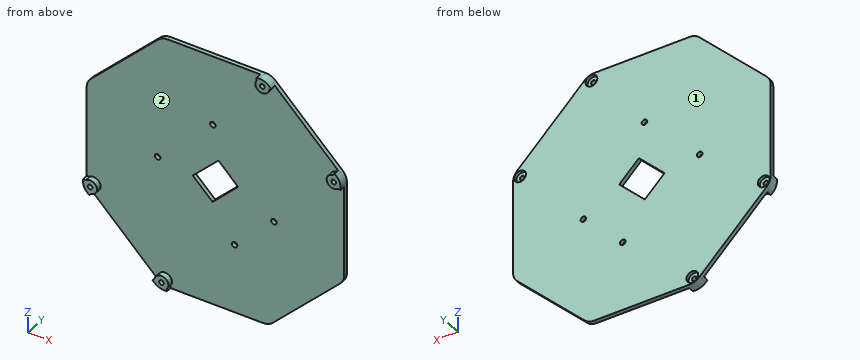
```python
from build123d import *

# Parameters (mm, degrees)
BOSS_EXTRUDE1_DEPTH                              = 3
BOSS_EXTRUDE3_DEPTH                              = 7
CBORE_FOR_M3_HEX_HEAD_MACHINE_SCREW1_D           = 3.4
CBORE_FOR_M3_HEX_HEAD_MACHINE_SCREW1_CBORE_D     = 8.4
CBORE_FOR_M3_HEX_HEAD_MACHINE_SCREW1_CBORE_DEPTH = 2.3
FILLET1_R                                        = 10
SKETCH23_R                                       = 2
CUT_EXTRUDE1_DEPTH                               = 131.843677004
CUT_EXTRUDE2_DEPTH                               = 131.843677004


with BuildPart() as part:
    # Sketch1 → Boss-Extrude1 (new body)
    with BuildSketch(Plane(origin=(0, 0, 0), x_dir=(1, 0, 0), z_dir=(0, 1, 0))):
        Polygon((92.387953251, -38.268343237), (92.387953251, 38.268343237), (38.268343237, 92.387953251), (-38.268343237, 92.387953251), (-92.387953251, 38.268343237), (-92.387953251, -38.268343237), (-38.268343237, -92.387953251), (38.268343237, -92.387953251), align=None)
    extrude(amount=BOSS_EXTRUDE1_DEPTH)

    # Sketch13 → Boss-Extrude3 (add)
    with BuildSketch(Plane(origin=(0, 3, 0), x_dir=(1, 0, 0), z_dir=(0, 1, 0))):
        with BuildLine():
            ThreePointArc((-90.387953251, 32.197275425), (-82.768555589, 34.283858263), (-86.68084647, 41.147022893))
            Line((-86.68084647, 41.147022893), (-88.095060032, 42.561236455))
            Line((-88.095060032, 42.561236455), (-92.387953251, 38.268343237))
            Line((-92.387953251, 38.268343237), (-92.387953251, 32.197275425))
            Line((-92.387953251, 32.197275425), (-90.387953251, 32.197275425))
        make_face()
        with BuildLine():
            Line((92.387953251, -32.197275425), (90.387953251, -32.197275425))
            ThreePointArc((90.387953251, -32.197275425), (82.768555589, -34.283858263), (86.68084647, -41.147022893))
            Line((86.68084647, -41.147022893), (88.095060032, -42.561236455))
            Line((88.095060032, -42.561236455), (92.387953251, -38.268343237))
            Line((92.387953251, -38.268343237), (92.387953251, -32.197275425))
        make_face()
        with BuildLine():
            Line((38.268343237, -92.387953251), (42.561236455, -88.095060032))
            Line((42.561236455, -88.095060032), (41.147022893, -86.68084647))
            ThreePointArc((41.147022893, -86.68084647), (34.283858263, -82.768555589), (32.197275425, -90.387953251))
            Line((32.197275425, -90.387953251), (32.197275425, -92.387953251))
            Line((32.197275425, -92.387953251), (38.268343237, -92.387953251))
        make_face()
        with BuildLine():
            ThreePointArc((-41.147022893, 86.68084647), (-34.283858263, 82.768555589), (-32.197275425, 90.387953251))
            Line((-32.197275425, 90.387953251), (-32.197275425, 92.387953251))
            Line((-32.197275425, 92.387953251), (-38.268343237, 92.387953251))
            Line((-38.268343237, 92.387953251), (-42.561236455, 88.095060032))
            Line((-42.561236455, 88.095060032), (-41.147022893, 86.68084647))
        make_face()
    extrude(amount=-BOSS_EXTRUDE3_DEPTH)

    # CBORE for M3 Hex Head Machine Screw1 (through all)
    with Locations(Plane(origin=(0, 3, 0), x_dir=(1, 0, 0), z_dir=(0, 1, 0))):
        with Locations((36.197275425, -87.387953251), (87.387953251, -36.197275425), (-36.197275425, 87.387953251), (-87.387953251, 36.197275425)):
            CounterBoreHole(CBORE_FOR_M3_HEX_HEAD_MACHINE_SCREW1_D / 2, CBORE_FOR_M3_HEX_HEAD_MACHINE_SCREW1_CBORE_D / 2, CBORE_FOR_M3_HEX_HEAD_MACHINE_SCREW1_CBORE_DEPTH)

    # Fillet1
    fillet1_edges = [part.edges().sort_by_distance(p)[0] for p in [
        (-92.387953251, 1.5, 38.268343237),
        (-92.387953251, -0.5, -38.268343237),
        (-38.268343237, -0.5, -92.387953251),
        (38.268343237, 1.5, -92.387953251),
        (92.387953251, 1.5, -38.268343237),
        (92.387953251, -0.5, 38.268343237),
        (38.268343237, -0.5, 92.387953251),
        (-38.268343237, 1.5, 92.387953251),
    ]]
    fillet(fillet1_edges, radius=FILLET1_R)

    # Sketch23 → Cut-Extrude1 (cut, through all)
    with BuildSketch(Plane(origin=(0, 3, 0), x_dir=(1, 0, 0), z_dir=(0, 1, 0))):
        with Locations(Location((-41.471812717, -1.87383297, 0), (0, 0, 270))):
            Circle(SKETCH23_R)
        with Locations(Location((13.682516216, 41.966787463, 0), (0, 0, 270))):
            Circle(SKETCH23_R)
        with Locations(Location((41.966787463, 13.682516216, 0), (0, 0, 270))):
            Circle(SKETCH23_R)
        with Locations(Location((-1.87383297, -41.471812717, 0), (0, 0, 270))):
            Circle(SKETCH23_R)
    extrude(amount=-CUT_EXTRUDE1_DEPTH, mode=Mode.SUBTRACT)

    # Sketch24 → Cut-Extrude2 (cut, through all)
    with BuildSketch(Plane(origin=(0, 3, 0), x_dir=(1, 0, 0), z_dir=(0, 1, 0))):
        Polygon((-16.263455967, 2.121320344), (-2.121320344, 16.263455967), (16.263455967, -2.121320344), (2.121320344, -16.263455967), align=None)
    extrude(amount=-CUT_EXTRUDE2_DEPTH, mode=Mode.SUBTRACT)


solid = part.part
```
Geometry check sheet. Reference: the model listing, model coordinates, mm. Face numbers are marked on the shaded views. A direction names the side the tool comes from. Give positions to 0.01 mm unless a question says otherwise; leave off trailing zeros. Loops run counter-clockwise (first coordinate to the right, second up) from the corner with the lowest first, then second, coordinate; pieces in that order, holes last. Notation, with made-up numbers: M 60.5,87.5 L 83.5,87.5 A9 cw 83.5,95.5 Z; hole C 54,-24.75 d1. An arc over 180 degrees is marked long. Write item = value, one per line.
(1) Sectioned sample at B-B, the plane y = -2.75. Record the cut outline in (x, z).
Answer below:
outline = M -92.39,-34.13 A10 ccw -89.46,-41.2 L -88.1,-42.56 L -86.68,-41.15 A5 ccw long -90.39,-32.2 L -92.39,-32.2 Z; M -42.56,-88.1 L -41.2,-89.46 A10 ccw -34.13,-92.39 L -32.2,-92.39 L -32.2,-90.39 A5 ccw long -41.15,-86.68 Z; M 32.2,90.39 A5 ccw long 41.15,86.68 L 42.56,88.1 L 41.2,89.46 A10 ccw 34.13,92.39 L 32.2,92.39 Z; M 86.68,41.15 A5 ccw long 90.39,32.2 L 92.39,32.2 L 92.39,34.13 A10 ccw 89.46,41.2 L 88.1,42.56 Z; hole C -87.39,-36.2 d3.4; hole C -36.2,-87.39 d3.4; hole C 36.2,87.39 d3.4; hole C 87.39,36.2 d3.4
(2) Gauge pin test, flat ends, axial feed: pin 1 Ø1.5 at (x, z) = (10.5, 64) entering from -Y; pin 2 Ø2 at (y, z) = (1, 42.5) entering from +X; pin 3 Ø2.5 at (x, z) = (-88.5, -36.5) entering from +Y; pin 4 Ø6.5 at (x, z) = (-87.39, -36.2) entering from -Y. Record the tip position at first contact, or that the pin passes through.
Answer below:
pin_1 = 0
pin_2 = 89.16
pin_3 = 0.7
pin_4 = -4
(3) Sectioned sample at C-C, the plane x = -24.5. Record the cut outline in (y, z).
Answer below:
outline = M 0,-92.39 L 3,-92.39 L 3,92.39 L 0,92.39 Z
(4) Tool access check on the marked faces 1 and 2. Record the directions out of +Z, -Z, +X, -X, +Y, -Y that give a thin tool (end or side, any length) a straight path to the whole face; none if there is none.
Answer below:
face_1 = +Z, -Z, +X, -X, +Y
face_2 = -Y
(5) Material ranges on line 1 (Z direction, x = -42, y = 0.75); line 2 (Y direction, x = 30, z = -80); line 3 (X direction, y = 2.25, z = 3), recorded low to high. Write a range as [from, to].
Answer below:
line_1 = [-88.66, -0.06], [3.8, 88.66]
line_2 = [0, 3]
line_3 = [-92.39, -43.12], [-39.82, -11.14], [15.38, 92.39]
(6) Sectioned sample at A-A, the plane x = 9.5. Record the cut outline in (y, z), plus the area to 3 significant figures.
Answer below:
outline = M 0,-92.39 L 3,-92.39 L 3,-4.64 L 0,-4.64 Z; M 0,8.88 L 3,8.88 L 3,92.39 L 0,92.39 Z
area = 514 mm2
(7) Sectioned sample at D-D, the plane z = 69.5. Record the cut outline in (x, y).
Answer below:
outline = M -61.16,0 L 61.16,0 L 61.16,3 L -61.16,3 Z
